Verification items for the finished model (mm, model axes). A direction names the side the tool comes from. Coordinates: 2 decimals unless noted, no trailing zeros. Loops run counter-clockwise (first coordinate to the right, second up) from the corner with the lowest first, then second, coordinate; pieces in that order, holes last. Notation, with made-up numbers: (36.5, 59) - (69.5, 59) arc R33 ccw to (69.5, 93) - close; hole circle Ø2 at (-3, -7.5). An arc over 180 degrees is marked (long way). One line per item, written item: value. Start each with the question number.
(1) Draft check along X on faces 4 (the face through (26, -10, 39)), 5 (the face through (6.53, 5.26, 39.44)), 6 (the face through (-10, -6, 39)), 7 (the face through (-8.2, 4, 39)). Enter one of: +X half, -X half, draft (parallel to the pull), parting line (faces both ways), or undercut.
(2) Set-up check for faces 1 (the face through (16, 8.2, 39)), 2 (the face through (20, -3.65, 39)), 3 (the face through (26, 10, 39)): record each of +Z, -Z, +X, -X, +Y, -Y from which the full face is reachable in a straight line by a thin tool's end or side.
(3) Section check B-B (y = 0). Record the boundary of the cut face in (x, z).
(4) Section check C-C (z = 50). Count the separate pieces of the cut face and the enclosed holes in it, plus the area to 3 significant figures.
(5) Gauge pin test, flat ends, axial feed: P1, Ø0.7, axis at x = 19.5, z = 55.5, coming from the +Y side; P2, Ø1.1, axis at y = 0, z = 34.5, coming from the -X side; P3, Ø2.5, axis at x = 0.5, z = 44.5, coming from the +Y side. Record the tip position at first contact, or that the pin passes through.
(6) Thickness scan on probe 1 along Y at (x, z) = (10, 15.5); probe 2 along Y at (x, z) = (20, 64); probe 3 along X at (y, z) = (3.5, 32). Record the ranges inside material, lowest first. Write a range as [from, to].
(7) Section check A-A (x = 20). Record the boundary of the cut face in (y, z).
```python
from build123d import *

# Parameters (mm, degrees)
CROQUIS3_R              = 2.15
SALIENTE_EXTRUIR1_DEPTH = 80


with BuildPart() as part:
    # Croquis3 → Saliente-Extruir1 (new body)
    with BuildSketch(Plane.XY):
        with BuildLine():
            Line((-2.574814133, 9.2), (-2.574814133, 8.5))
            ThreePointArc((-2.574814133, 8.5), (-2.662682099, 8.287867966), (-2.874814133, 8.2))
            Line((-2.874814133, 8.2), (-5.044814133, 8.2))
            ThreePointArc((-5.044814133, 8.2), (-5.765448465, 7.718473047), (-5.596326761, 6.868426051))
            Line((-5.596326761, 6.868426051), (-3.255673209, 4.528032719))
            ThreePointArc((-3.255673209, 4.528032719), (-2.282627587, 3.878186348), (-1.135, 3.65))
            Line((-1.135, 3.65), (1.135, 3.65))
            ThreePointArc((1.135, 3.65), (2.282627587, 3.878186348), (3.255673209, 4.528032719))
            Line((3.255673209, 4.528032719), (5.596326761, 6.868426051))
            ThreePointArc((5.596326761, 6.868426051), (5.765448465, 7.718473047), (5.044814133, 8.2))
            Line((5.044814133, 8.2), (2.874814133, 8.2))
            ThreePointArc((2.874814133, 8.2), (2.662682099, 8.287867966), (2.574814133, 8.5))
            Line((2.574814133, 8.5), (2.574814133, 9.2))
            ThreePointArc((2.574814133, 9.2), (2.809128708, 9.765685425), (3.374814133, 10))
            Line((3.374814133, 10), (16.625185867, 10))
            ThreePointArc((16.625185867, 10), (17.190871292, 9.765685425), (17.425185867, 9.2))
            Line((17.425185867, 9.2), (17.425185867, 8.5))
            ThreePointArc((17.425185867, 8.5), (17.337317901, 8.287867966), (17.125185867, 8.2))
            Line((17.125185867, 8.2), (14.955185867, 8.2))
            ThreePointArc((14.955185867, 8.2), (14.234551535, 7.718473047), (14.403673239, 6.868426051))
            Line((14.403673239, 6.868426051), (16.744326791, 4.528032719))
            ThreePointArc((16.744326791, 4.528032719), (17.717372413, 3.878186348), (18.865, 3.65))
            Line((18.865, 3.65), (21.135, 3.65))
            ThreePointArc((21.135, 3.65), (22.282627587, 3.878186348), (23.255673209, 4.528032719))
            Line((23.255673209, 4.528032719), (25.596326761, 6.868426051))
            ThreePointArc((25.596326761, 6.868426051), (25.765448465, 7.718473047), (25.044814133, 8.2))
            Line((25.044814133, 8.2), (22.874814133, 8.2))
            ThreePointArc((22.874814133, 8.2), (22.662682099, 8.287867966), (22.574814133, 8.5))
            Line((22.574814133, 8.5), (22.574814133, 9.2))
            ThreePointArc((22.574814133, 9.2), (22.809128708, 9.765685425), (23.374814133, 10))
            Line((23.374814133, 10), (28, 10))
            ThreePointArc((28, 10), (29.414213562, 9.414213562), (30, 8))
            Line((30, 8), (30, 3.374814133))
            ThreePointArc((30, 3.374814133), (29.765685425, 2.809128708), (29.2, 2.574814133))
            Line((29.2, 2.574814133), (28.5, 2.574814133))
            ThreePointArc((28.5, 2.574814133), (28.287867966, 2.662682099), (28.2, 2.874814133))
            Line((28.2, 2.874814133), (28.2, 5.044814133))
            ThreePointArc((28.2, 5.044814133), (27.718473047, 5.765448465), (26.868426051, 5.596326761))
            Line((26.868426051, 5.596326761), (24.528032719, 3.255673209))
            ThreePointArc((24.528032719, 3.255673209), (23.878186348, 2.282627587), (23.65, 1.135))
            Line((23.65, 1.135), (23.65, -1.135))
            ThreePointArc((23.65, -1.135), (23.878186348, -2.282627587), (24.528032719, -3.255673209))
            Line((24.528032719, -3.255673209), (26.868426051, -5.596326761))
            ThreePointArc((26.868426051, -5.596326761), (27.718473047, -5.765448465), (28.2, -5.044814133))
            Line((28.2, -5.044814133), (28.2, -2.874814133))
            ThreePointArc((28.2, -2.874814133), (28.287867966, -2.662682099), (28.5, -2.574814133))
            Line((28.5, -2.574814133), (29.2, -2.574814133))
            ThreePointArc((29.2, -2.574814133), (29.765685425, -2.809128708), (30, -3.374814133))
            Line((30, -3.374814133), (30, -8))
            ThreePointArc((30, -8), (29.414213562, -9.414213562), (28, -10))
            Line((28, -10), (23.374814133, -10))
            ThreePointArc((23.374814133, -10), (22.809128708, -9.765685425), (22.574814133, -9.2))
            Line((22.574814133, -9.2), (22.574814133, -8.5))
            ThreePointArc((22.574814133, -8.5), (22.662682099, -8.287867966), (22.874814133, -8.2))
            Line((22.874814133, -8.2), (25.044814133, -8.2))
            ThreePointArc((25.044814133, -8.2), (25.765448465, -7.718473047), (25.596326761, -6.868426051))
            Line((25.596326761, -6.868426051), (23.255673209, -4.528032719))
            ThreePointArc((23.255673209, -4.528032719), (22.282627587, -3.878186348), (21.135, -3.65))
            Line((21.135, -3.65), (18.865, -3.65))
            ThreePointArc((18.865, -3.65), (17.717372413, -3.878186348), (16.744326791, -4.528032719))
            Line((16.744326791, -4.528032719), (14.403673239, -6.868426051))
            ThreePointArc((14.403673239, -6.868426051), (14.234551535, -7.718473047), (14.955185867, -8.2))
            Line((14.955185867, -8.2), (17.125185867, -8.2))
            ThreePointArc((17.125185867, -8.2), (17.337317901, -8.287867966), (17.425185867, -8.5))
            Line((17.425185867, -8.5), (17.425185867, -9.2))
            ThreePointArc((17.425185867, -9.2), (17.190871292, -9.765685425), (16.625185867, -10))
            Line((16.625185867, -10), (3.374814133, -10))
            ThreePointArc((3.374814133, -10), (2.809128708, -9.765685425), (2.574814133, -9.2))
            Line((2.574814133, -9.2), (2.574814133, -8.5))
            ThreePointArc((2.574814133, -8.5), (2.662682099, -8.287867966), (2.874814133, -8.2))
            Line((2.874814133, -8.2), (5.044814133, -8.2))
            ThreePointArc((5.044814133, -8.2), (5.765448465, -7.718473047), (5.596326761, -6.868426051))
            Line((5.596326761, -6.868426051), (3.255673209, -4.528032719))
            ThreePointArc((3.255673209, -4.528032719), (2.282627587, -3.878186348), (1.135, -3.65))
            Line((1.135, -3.65), (-1.135, -3.65))
            ThreePointArc((-1.135, -3.65), (-2.282627587, -3.878186348), (-3.255673209, -4.528032719))
            Line((-3.255673209, -4.528032719), (-5.596326761, -6.868426051))
            ThreePointArc((-5.596326761, -6.868426051), (-5.765448465, -7.718473047), (-5.044814133, -8.2))
            Line((-5.044814133, -8.2), (-2.874814133, -8.2))
            ThreePointArc((-2.874814133, -8.2), (-2.662682099, -8.287867966), (-2.574814133, -8.5))
            Line((-2.574814133, -8.5), (-2.574814133, -9.2))
            ThreePointArc((-2.574814133, -9.2), (-2.809128708, -9.765685425), (-3.374814133, -10))
            Line((-3.374814133, -10), (-8, -10))
            ThreePointArc((-8, -10), (-9.414213562, -9.414213562), (-10, -8))
            Line((-10, -8), (-10, -3.374814133))
            ThreePointArc((-10, -3.374814133), (-9.765685425, -2.809128708), (-9.2, -2.574814133))
            Line((-9.2, -2.574814133), (-8.5, -2.574814133))
            ThreePointArc((-8.5, -2.574814133), (-8.287867966, -2.662682099), (-8.2, -2.874814133))
            Line((-8.2, -2.874814133), (-8.2, -5.044814133))
            ThreePointArc((-8.2, -5.044814133), (-7.718473047, -5.765448465), (-6.868426051, -5.596326761))
            Line((-6.868426051, -5.596326761), (-4.528032719, -3.255673209))
            ThreePointArc((-4.528032719, -3.255673209), (-3.878186348, -2.282627587), (-3.65, -1.135))
            Line((-3.65, -1.135), (-3.65, 1.135))
            ThreePointArc((-3.65, 1.135), (-3.878186348, 2.282627587), (-4.528032719, 3.255673209))
            Line((-4.528032719, 3.255673209), (-6.868426051, 5.596326761))
            ThreePointArc((-6.868426051, 5.596326761), (-7.718473047, 5.765448465), (-8.2, 5.044814133))
            Line((-8.2, 5.044814133), (-8.2, 2.874814133))
            ThreePointArc((-8.2, 2.874814133), (-8.287867966, 2.662682099), (-8.5, 2.574814133))
            Line((-8.5, 2.574814133), (-9.2, 2.574814133))
            ThreePointArc((-9.2, 2.574814133), (-9.765685425, 2.809128708), (-10, 3.374814133))
            Line((-10, 3.374814133), (-10, 8))
            ThreePointArc((-10, 8), (-9.414213562, 9.414213562), (-8, 10))
            Line((-8, 10), (-3.374814133, 10))
            ThreePointArc((-3.374814133, 10), (-2.809128708, 9.765685425), (-2.574814133, 9.2))
        make_face()
        Circle(CROQUIS3_R, mode=Mode.SUBTRACT)
        with Locations((20, 0)):
            Circle(CROQUIS3_R, mode=Mode.SUBTRACT)
        with BuildLine():
            Line((4.528394658, 3.25516976), (8.586400769, 7.314749345))
            ThreePointArc((8.586400769, 7.314749345), (9.234932122, 7.748324734), (10, 7.900809736))
            ThreePointArc((10, 7.900809736), (10.765067878, 7.748324734), (11.413599231, 7.314749345))
            Line((11.413599231, 7.314749345), (15.471605342, 3.25516976))
            ThreePointArc((15.471605342, 3.25516976), (16.121559892, 2.282196395), (16.349873833, 1.134594184))
            Line((16.349873833, 1.134594184), (16.349873833, -1.134594184))
            ThreePointArc((16.349873833, -1.134594184), (16.121559892, -2.282196395), (15.471605342, -3.25516976))
            Line((15.471605342, -3.25516976), (11.413599231, -7.314749345))
            ThreePointArc((11.413599231, -7.314749345), (10, -7.900441833), (8.586400769, -7.314749345))
            Line((8.586400769, -7.314749345), (4.528394658, -3.25516976))
            ThreePointArc((4.528394658, -3.25516976), (3.878440108, -2.282196395), (3.650126167, -1.134594184))
            Line((3.650126167, -1.134594184), (3.650126167, 1.134594184))
            ThreePointArc((3.650126167, 1.134594184), (3.878440108, 2.282196395), (4.528394658, 3.25516976))
        make_face(mode=Mode.SUBTRACT)
    extrude(amount=SALIENTE_EXTRUIR1_DEPTH)


solid = part.part
```
Responses:
1. face 4: draft
1. face 5: undercut
1. face 6: -X half
1. face 7: undercut
2. face 1: +Z, -Z
2. face 2: +Z, -Z, -Y
2. face 3: +Z, -Z, +X, -X, +Y
3. outline: (-3.65, 0) - (-2.15, 0) - (-2.15, 80) - (-3.65, 80) - close; (2.15, 0) - (3.65, 0) - (3.65, 80) - (2.15, 80) - close; (16.35, 0) - (17.85, 0) - (17.85, 80) - (16.35, 80) - close; (22.15, 0) - (23.65, 0) - (23.65, 80) - (22.15, 80) - close
4. separate pieces: 1
4. enclosed holes: 3
4. area: 329 mm²
5. P1: stops at y = 3.65
5. P2: stops at x = -3.65
5. P3: stops at y = 3.71
6. probe 1: y = [-10, -7.9], [7.9, 10]
6. probe 2: y = [-3.65, -2.15], [2.15, 3.65]
6. probe 3: x = [-10, -8.2], [-4.77, 4.77], [15.23, 24.77], [28.2, 30]
7. outline: (-3.65, 0) - (-2.15, 0) - (-2.15, 80) - (-3.65, 80) - close; (2.15, 0) - (3.65, 0) - (3.65, 80) - (2.15, 80) - close
